from build123d import *

# Parameters (mm, degrees)
BOSS_EXTRUDE1_DEPTH     = 19
SKETCH2_R               = 15
BOSS_EXTRUDE2_DEPTH     = 8
SKETCH4_R               = 28
SKETCH4_R_2             = 18
CUT_EXTRUDE_THIN1_DEPTH = 0.6
CUT_EXTRUDE1_REACH      = 29
SKETCH5_R               = 11
CUT_EXTRUDE2_START      = -15
CUT_EXTRUDE2_DEPTH      = 4.349296
CIRPATTERN1_COUNT       = 6
CHAMFER1_SIZE           = 1


with BuildPart() as part:
    # Sketch1 → Boss-Extrude1 (new body)
    with BuildSketch(Plane.XY):
        Polygon((20.784609691, 0), (10.392304845, 18), (-10.392304845, 18), (-20.784609691, 0), (-10.392304845, -18), (10.392304845, -18), align=None)
    extrude(amount=BOSS_EXTRUDE1_DEPTH)

    # Sketch2 → Boss-Extrude2 (add)
    with BuildSketch(Plane.XY.offset(19)):
        Circle(SKETCH2_R)
    extrude(amount=BOSS_EXTRUDE2_DEPTH)

    # Sketch3 → Cut-Revolve1 (revolve, cut)
    with BuildSketch(Plane(origin=(0, 0, 0), x_dir=(0, 0, -1), z_dir=(1, 0, 0))):
        Polygon((-19, 15), (-19, 25.977792564), (-12.661968508, 25.977792564), align=None)
    revolve(axis=Axis((0, 0, -102.328960849), (0, 0, 1)), mode=Mode.SUBTRACT)

    # Sketch4 → Cut-Extrude-Thin1 (cut)
    with BuildSketch(Plane(origin=(0, 0, 0), x_dir=(-1, 0, 0), z_dir=(0, 0, -1))):
        Circle(SKETCH4_R)
        Circle(SKETCH4_R_2, mode=Mode.SUBTRACT)
    extrude(amount=-CUT_EXTRUDE_THIN1_DEPTH, mode=Mode.SUBTRACT)

    # Sketch5 → Cut-Extrude1 (cut, up to next)
    with BuildSketch(Plane.XY.offset(27), mode=Mode.PRIVATE) as cut_extrude1_sk1:
        Circle(SKETCH5_R)
    cut_extrude1_tool1 = extrude(cut_extrude1_sk1.sketch, amount=-CUT_EXTRUDE1_REACH, mode=Mode.PRIVATE) & part.part
    add(cut_extrude1_tool1.solids().sort_by_distance((0, 0, 27))[0], mode=Mode.SUBTRACT)

    # Sketch6 → Cut-Extrude2 (cut)
    with BuildSketch(Plane(origin=(0, 0, 0), x_dir=(1, 0, 0), z_dir=(0, 1, 0)).offset(CUT_EXTRUDE2_START)):
        with BuildLine():
            Line((-2.75, -21.75), (-2.75, -27))
            Line((-2.75, -27), (2.75, -27))
            Line((2.75, -27), (2.75, -21.75))
            ThreePointArc((2.75, -21.75), (0, -19), (-2.75, -21.75))
        make_face()
    cut_extrude2 = extrude(amount=CUT_EXTRUDE2_DEPTH, mode=Mode.SUBTRACT)

    # CirPattern1: Cut-Extrude2 ×6 about axis
    cirpattern1_axis = Axis((0, 0, 0), (0, 0, 1))
    for i in range(1, CIRPATTERN1_COUNT):
        add(cut_extrude2.rotate(cirpattern1_axis, i * 360 / CIRPATTERN1_COUNT), mode=Mode.SUBTRACT)

    # Chamfer1
    chamfer1_edges = [part.edges().sort_by_distance(p)[0] for p in [
        (-11, 0, 0),
        (5.5, -9.526279442, 27),
        (10.899233565, 1.485499137, 27),
        (5.5, 9.526279442, 27),
        (-5.5, 9.526279442, 27),
        (-11, 0, 27),
        (-5.5, -9.526279442, 27),
    ]]
    chamfer(chamfer1_edges, length=CHAMFER1_SIZE)


solid = part.part
Could you check a few things on this model? Use its own coordinates, in mm. A direction names the side the tool comes from. Round coordinates to 2 decimals unless told otherwise and drop trailing zeros. Write each loop counter-clockwise with the first axis right and the second up, starting at its lowest first coordinate (ties: lowest second). Pieces come first, ordered by that corner, then holes. Notation, with made-up numbers: (-3, -26.75) -> (26, -26.75) arc R33 ccw to (26, 7.25) -> close; hole circle Ø8 at (49.25, 54.5). An arc over 180 degrees is marked (long way). Use a Markdown table: item, result.
1. Please list where these lines run through material, in increasing order: probe 1 along Y at (x, z) = (0, 11.25); probe 2 along X at (y, z) = (0, 6.5); probe 3 along X at (y, z) = (0, 19.25).
Answer key:
| item | result |
|---|---|
| probe 1 | y = -18 to -11, 11 to 18 |
| probe 2 | x = -20.78 to -11, 11 to 20.78 |
| probe 3 | x = -15 to -11, 11 to 15 |
2. Which directions (+Z, -Z, +X, -X, +Y, -Y) give clear straight access to the entire face, cutting with the end or side of a thin tool? Please do faces 1 (the face through (-5.657, 9.892, 26.396)), 2 (the face through (-2.75, 13, 24)), 3 (the face through (15.661, 8.874, 8.817)), 4 (the face through (-7, -11, 27)), 5 (the face through (-15, 0, 23)).
Answer key:
| item | result |
|---|---|
| face 1 | +Z |
| face 2 | +Z, +Y, -Y |
| face 3 | +Z, -Z, +X, +Y |
| face 4 | +Z, +X, -X, +Y, -Y |
| face 5 | +Z, -X |
3. For pin 1 Ø10 at (y, z) = (8.5, 17.5) entering from -X; pin 2 Ø20 at (x, y) = (0, 0) entering from +Z; pin 3 Ø4 at (x, y) = (18, 2.5) entering from -Z; pin 4 Ø1.5 at (y, z) = (-13.5, 23.5) entering from +X, each with a flat end and sliding along its axis, tell me the tip position at first contact or that it passes through.
Answer key:
| item | result |
|---|---|
| pin 1 | stops at x = -18.72 |
| pin 2 | passes through |
| pin 3 | stops at z = 0 |
| pin 4 | stops at x = 7.9 |
4. We'd pull the mould along X, two halves only. Please class faces 6 (the face through (-15.661, -8.874, 8.817)), 7 (the face through (-5.74, -9.85, 26.4)), 8 (the face through (9.647, 8.745, 24.412)): +X half, -X half, draft (parallel to the pull), parting line (faces both ways), or undercut.
Answer key:
| item | result |
|---|---|
| face 6 | -X half |
| face 7 | undercut |
| face 8 | +X half |
5. If we section it at A-A (z = 5): List the corners of the cut face in (x, y) for me.
Answer key:
| item | result |
|---|---|
| outline | (-20.78, 0) -> (-10.39, -18) -> (10.39, -18) -> (20.78, 0) -> (10.39, 18) -> (-10.39, 18) -> close; hole circle Ø22 at (0, 0) |
